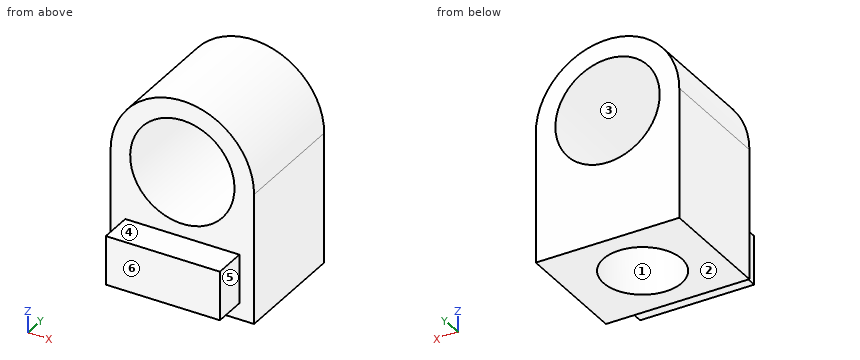
from build123d import *

# Parameters (mm, degrees)
SKETCH1_R           = 8
BOSS_EXTRUDE1_DEPTH = 18
SKETCH2_R           = 6
CUT_EXTRUDE1_DEPTH  = 10
SKETCH4_W           = 17.5
SKETCH4_H           = 7.5
BOSS_EXTRUDE3_DEPTH = 5


with BuildPart() as part:
    # Sketch1 → Boss-Extrude1 (new body)
    with BuildSketch(Plane(origin=(0, 0, 0), x_dir=(1, 0, 0), z_dir=(0, 1, 0))):
        with BuildLine():
            Line((-11, 0), (-11, 20))
            Line((-11, 20), (11, 20))
            Line((11, 20), (11, 0))
            ThreePointArc((11, 0), (0, -11), (-11, 0))
        make_face()
        with Locations(Location((0, 0, 0), (0, 0, 270))):
            Circle(SKETCH1_R, mode=Mode.SUBTRACT)
    extrude(amount=BOSS_EXTRUDE1_DEPTH)

    # Sketch2 → Cut-Extrude1 (cut)
    with BuildSketch(Plane(origin=(0, 0, -20), x_dir=(-1, 0, 0), z_dir=(0, 0, -1))):
        with Locations((0, 9)):
            Circle(SKETCH2_R)
    extrude(amount=-CUT_EXTRUDE1_DEPTH, mode=Mode.SUBTRACT)

    # Sketch4 → Boss-Extrude3 (add)
    with BuildSketch(Plane.XZ):
        with Locations((0, -13.75)):
            Rectangle(SKETCH4_W, SKETCH4_H)
    extrude(amount=BOSS_EXTRUDE3_DEPTH)


solid = part.part
Check sheet for the modelled part. Datum: model origin and axes. Units: mm. Face numbers are marked on the shaded views. A direction names the side the tool comes from. Round coordinates to 2 decimals unless told otherwise and drop trailing zeros. Loops run counter-clockwise (first coordinate to the right, second up) from the corner with the lowest first, then second, coordinate; pieces in that order, holes last.
1. Set-up check for the marked faces 5 and 6: record each of +Z, -Z, +X, -X, +Y, -Y from which the full face is reachable in a straight line by a thin tool's end or side.
2. Sectioned sample at A-A on z = -11. Record the boundary of the cut face in (x, y), and give its area (3 significant figures).
3. Sectioned sample at B-B on x = 0. Record the boundary of the cut face in (y, z).
4. Sectioned sample at D-D on z = -1. Record the boundary of the cut face in (x, y).
5. Gauge pin test, flat ends, axial feed: pin 1 Ø2.5 at (y, z) = (-2.5, -13) entering from -X; pin 2 Ø1 at (x, y) = (4, 8.5) entering from -Z; pin 3 Ø2 at (y, z) = (13, 6) entering from +X. Record the tip position at first contact, or that the pin passes through.
6. Scan lines: probe 1 along X at (y, z) = (8.5, 0); probe 2 along Y at (x, z) = (0, -16); probe 3 along Z at (x, y) = (-0.25, 1.5). Record each from-to range of solid material in increasing order.
7. Sectioned sample at C-C on y = 9. Record the boundary of the cut face in (x, z).
8. Mould release check, pull along Z, two halves, no side actions. Record for the marked faces 1, 2, 3 and 4: released by +Z, released by -Z, zero draft, split by the parting line, or undercut.
Recorded:
1. face 5: +Z, -Z, +X, -Y
1. face 6: +Z, -Z, +X, -X, -Y
2. outline: (-11, 0) - (-8.75, 0) - (-8.75, -5) - (8.75, -5) - (8.75, 0) - (11, 0) - (11, 18) - (-11, 18) - close; hole circle Ø12 at (0, 9)
2. area: 370 mm2
3. outline: (-5, -17.5) - (0, -17.5) - (0, -20) - (3, -20) - (3, -10) - (15, -10) - (15, -20) - (18, -20) - (18, -8) - (0, -8) - (0, -10) - (-5, -10) - close; (0, 8) - (18, 8) - (18, 11) - (0, 11) - close
4. outline: (-11, 0) - (-7.94, 0) - (-7.94, 18) - (-11, 18) - close; (7.94, 0) - (11, 0) - (11, 18) - (7.94, 18) - close
5. pin 1: stops at x = -8.75
5. pin 2: stops at z = -10
5. pin 3: stops at x = 9.8
6. probe 1: x = -11 to -8, 8 to 11
6. probe 2: y = -5 to 3, 15 to 18
6. probe 3: z = -20 to -8, 8 to 11
7. outline: (-11, -20) - (-6, -20) - (-6, -10) - (6, -10) - (6, -20) - (11, -20) - (11, 0) arc R11 ccw to (-11, 0) - close; hole circle Ø16 at (0, 0)
8. face 1: zero draft
8. face 2: released by -Z
8. face 3: undercut
8. face 4: released by +Z
